from build123d import *

# Parameters (mm, degrees)
F1_DEPTH = 40
F2_R     = 3.25
F3_DEPTH = 104.501
F5_DEPTH = 40.501
F6_R     = 10
F7_R     = 4.99999
F8_R     = 5


# Not quite as in the source:
# - a fillet or chamfer is up to 0.001 mm smaller than in the source, because OpenCascade refuses the exact size


with BuildPart() as f1:
    # F0 (on Top) → F1 (new body)
    with BuildSketch(Plane.XY):
        Polygon((0, 66), (0, 0), (9.5, 0), (9.5, 25.5), (104.5, 25.5), (104.5, 40.5), (9.5, 40.5), (9.5, 66), align=None)
    extrude(amount=F1_DEPTH)

    # F2 (on face) → F3 (cut, through all)
    with BuildSketch(Plane(origin=(0, 0, 0), x_dir=(0, -1, 0), z_dir=(-1, 0, 0))):
        with Locations((-56, 20)):
            Circle(F2_R)
        with Locations((-10, 20)):
            Circle(F2_R)
    extrude(amount=-F3_DEPTH, mode=Mode.SUBTRACT)

    # F4 (on face) → F5 (cut, through all)
    with BuildSketch(Plane.XZ.offset(-25.5)):
        with BuildLine():
            Line((65.5, 35), (91.5, 35))
            ThreePointArc((91.5, 35), (78.5, 48), (65.5, 35))
        make_face()
        with BuildLine():
            ThreePointArc((65.5, 35), (78.5, 22), (91.5, 35))
            Line((91.5, 35), (65.5, 35))
        make_face()
        with BuildLine():
            ThreePointArc((65.5, 35), (78.5, 48), (91.5, 35))
            Line((91.5, 35), (91.5, 50.4635125536))
            Line((91.5, 50.4635125536), (65.5, 50.4635125536))
            Line((65.5, 50.4635125536), (65.5, 35))
        make_face()
    extrude(amount=-F5_DEPTH, mode=Mode.SUBTRACT)

    # F6
    f6_edges = [f1.edges().sort_by_distance(p)[0] for p in [
        (9.5, 25.5, 20),
        (9.5, 40.5, 20),
    ]]
    fillet(f6_edges, radius=F6_R)

    # F7 (radius 5 in the source; OpenCascade refuses exactly that, so slightly less here)
    f7_edges = [f1.edges().sort_by_distance(p)[0] for p in [
        (65.5, 33, 40),
        (91.5, 33, 40),
    ]]
    fillet(f7_edges, radius=F7_R)

    # F8
    f8_edges = [f1.edges().sort_by_distance(p)[0] for p in [
        (104.5, 33, 40),
    ]]
    fillet(f8_edges, radius=F8_R)


solid = f1.part
Could you check a few things on this model? Use its own coordinates, in mm. A direction names the side the tool comes from. Coordinates: 2 decimals unless noted, no trailing zeros. Loops run counter-clockwise (first coordinate to the right, second up) from the corner with the lowest first, then second, coordinate; pieces in that order, holes last.
1. I need wall thicknesses on L1, parallel to Z at x = 2.75, y = 10; L2, parallel to X at y = 5, z = 11; L3, parallel to Y at x = 31, z = 7. Which ranges of each line are inside material? Lowest first, please.
2. We'd pull the mould along Z, two halves only. Please class faces 6 (the face through (40, 33, 0)), 7 (the face through (4.684, 12.579, 18.022)), 8 (the face through (61, 25.5, 20)), 9 (the face through (103.07, 33.11, 38.5)): released by +Z, released by -Z, zero draft, split by the parting line, or undercut.
3. Imagine slicing it at D-D (y = 44.5). Please give me the cut outline in (x, z), and give its area (3 significant figures).
4. For faces 1 (the face through (23, 33, 40)), 2 (the face through (64, 32.89, 38.57)), 3 (the face through (5, 66, 20)), 4 (the face through (9.5, 60, 20)), 5 (the face through (9.5, 6, 20)), which set-ups out of +Z, -Z, +X, -X, +Y, -Y let a thin tool reach every point of the face, with its end or its side?
5. Imagine slicing it at A-A (z = 20). Please give me the cut outline in (x, y), and give its area (3 significant figures).
6. For P1, Ø1.5, axis at x = 81.5, y = 38, coming from the +Z side; P2, Ø1.5, axis at x = 26.5, z = 23.5, coming from the +Y side; P3, Ø4.5, axis at y = 5.5, z = 10.5, coming from the +X side, each with a flat end and sliding along its axis, tell me the tip position at first contact or that it passes through.
7. Imagine slicing it at B-B (y = 10). Please give me the cut outline in (x, z).
8. Imagine slicing it at C-C (x = 78.5). Please give me the cut outline in (y, z), and give its area (3 significant figures).
Computed values:
1. L1: z = 0 to 16.75, 23.25 to 40
1. L2: x = 0 to 9.5
1. L3: y = 25.5 to 40.5
2. face 6: released by -Z
2. face 7: undercut
2. face 8: zero draft
2. face 9: released by +Z
3. outline: (0, 0) - (11.5, 0) - (11.5, 40) - (0, 40) - close
3. area: 460 mm2
4. face 1: +Z, +X, -X, +Y, -Y
4. face 2: +Z, +Y, -Y
4. face 3: +Z, -Z, +X, -X, +Y
4. face 4: +Z, -Z, +X, +Y
4. face 5: +Z, -Z, +X, -Y
5. outline: (0, 0) - (9.5, 0) - (9.5, 6.75) - (0, 6.75) - close; (0, 13.25) - (9.5, 13.25) - (9.5, 15.5) arc R10 cw to (19.5, 25.5) - (104.5, 25.5) - (104.5, 40.5) - (19.5, 40.5) arc R10 cw to (9.5, 50.5) - (9.5, 52.75) - (0, 52.75) - close; (0, 59.25) - (9.5, 59.25) - (9.5, 66) - (0, 66) - close
5. area: 1,970 mm2
6. P1: stops at z = 22.55
6. P2: stops at y = 40.5
6. P3: stops at x = 9.5
7. outline: (0, 0) - (9.5, 0) - (9.5, 16.75) - (0, 16.75) - close; (0, 23.25) - (9.5, 23.25) - (9.5, 40) - (0, 40) - close
8. outline: (25.5, 0) - (40.5, 0) - (40.5, 22) - (25.5, 22) - close
8. area: 330 mm2
